The figure shows three views and two pictorial views of one solid part (mm, origin at its lowest corner). Answer the questions. Round coordinates to 2 decimals unless told otherwise and drop trailing zeros. Order: outer loops, then holes, each group sorted by start corner. A loop starts at its lowest first (then second) coordinate and runs counter-clockwise, first axis right, second up. Notation, with made-up numbers: (-23.5, -1.75) -> (4.5, -1.75) arc R24 ccw to (4.5, 37.25) -> close; hole circle Ø6 at (31.25, 18). An arc over 180 degrees is marked (long way). One line per item, written item: value. Start each with the question number.
1. Section A-A (z = 6) is taken. Give the vertices of the cut face in (x, y).
2. Section B-B (x = 4) is taken. Give the vertices of the cut face in (y, z).
3. The mould has two halves that part along X. Classify the marked faces 1, 2, 3 and 4: released by +X, released by -X, zero draft, split by the parting line, or undercut.
4. Consider line 1 (Y direction, x = 4, z = 4.25); line 2 (X direction, y = 4.5, z = 1); line 3 (X direction, y = 4.25, z = 11.75). Determine where each line is inside the solid, lowest interval first.
5. Section D-D (z = 16.5) is taken. Give the vertices of the cut face in (x, y), then the cut area to 3 significant figures.
6. Flat-ended cylindrical pins translate along their axes: pin 1 Ø10 at (x, y) = (21, 7.5) entering from -Z; pin 2 Ø1 at (x, y) = (10, 11) entering from -Z; pin 3 Ø2 at (x, z) = (15.5, 8.5) entering from +Y. Find the tip coordinate at first contact, or state that the pin passes through.
7. Section C-C (y = 16) is taken. Give the vertices of the cut face in (x, z), then the cut area to 3 significant figures.
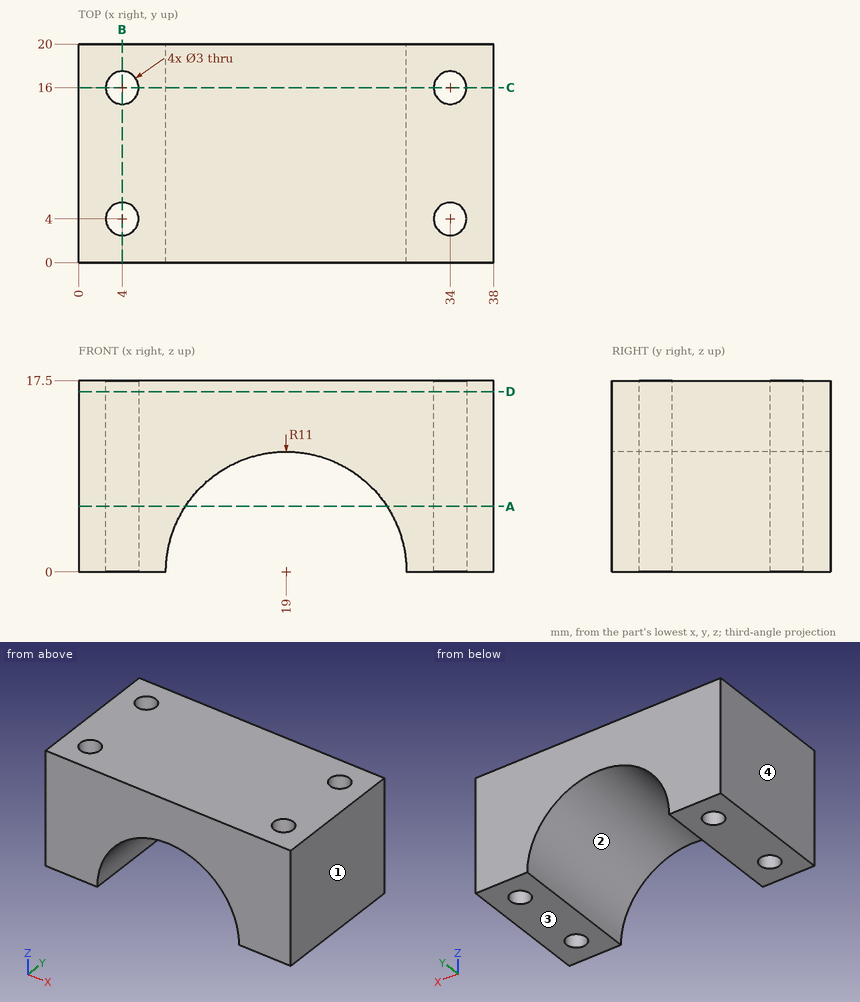
Answer:
1. outline: (0, 0) -> (9.78, 0) -> (9.78, 20) -> (0, 20) -> close; (28.22, 0) -> (38, 0) -> (38, 20) -> (28.22, 20) -> close; hole circle Ø3 at (4, 4); hole circle Ø3 at (4, 16); hole circle Ø3 at (34, 4); hole circle Ø3 at (34, 16)
2. outline: (0, 0) -> (2.5, 0) -> (2.5, 17.5) -> (0, 17.5) -> close; (5.5, 0) -> (14.5, 0) -> (14.5, 17.5) -> (5.5, 17.5) -> close; (17.5, 0) -> (20, 0) -> (20, 17.5) -> (17.5, 17.5) -> close
3. face 1: released by +X
3. face 2: undercut
3. face 3: zero draft
3. face 4: released by -X
4. line 1: 0 to 2.5, 5.5 to 14.5, 17.5 to 20
4. line 2: 0 to 2.59, 5.41 to 8.05, 29.95 to 32.59, 35.41 to 38
4. line 3: 0 to 2.52, 5.48 to 32.52, 35.48 to 38
5. outline: (0, 0) -> (38, 0) -> (38, 20) -> (0, 20) -> close; hole circle Ø3 at (4, 4); hole circle Ø3 at (4, 16); hole circle Ø3 at (34, 4); hole circle Ø3 at (34, 16)
5. area: 732 mm^2
6. pin 1: z = 8.49
6. pin 2: z = 5.55
6. pin 3: through
7. outline: (0, 0) -> (2.5, 0) -> (2.5, 17.5) -> (0, 17.5) -> close; (5.5, 0) -> (8, 0) arc R11 cw to (30, 0) -> (32.5, 0) -> (32.5, 17.5) -> (5.5, 17.5) -> close; (35.5, 0) -> (38, 0) -> (38, 17.5) -> (35.5, 17.5) -> close
7. area: 370 mm^2
